Part model, mm, in its own coordinate system. Give positions to 0.01 mm unless a question says otherwise; leave off trailing zeros. Write each loop counter-clockwise with the first axis right and the second up, starting at its lowest first coordinate (ties: lowest second). Pieces come first, ordered by that corner, then holes. Notation, with made-up numbers: (11, 30) - (26, 30) arc R24 cw to (26, 66) - close; hole circle Ø11 at (22, 23.25). An arc over 180 degrees is marked (long way). Answer as a JSON object with one key per item and string values. Group by question number.
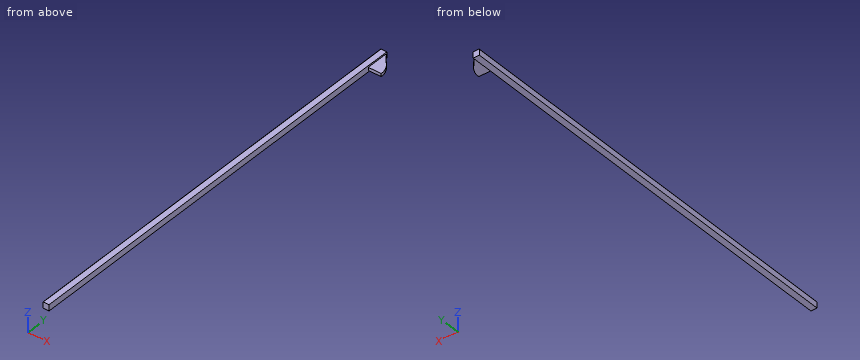
```python
from build123d import *

# Parameters (mm, degrees)
BOSS_EXTRUDE1_DEPTH = 0.220347005
SKETCH2_W           = 0.335173503
SKETCH2_H           = 31
BOSS_EXTRUDE2_DEPTH = 0.45
SKETCH3_W           = 0.45
SKETCH3_H           = 31
BOSS_EXTRUDE3_DEPTH = 0.114826497
FILLET1_R           = 0.025


with BuildPart() as part:
    # Sketch1 → Boss-Extrude1 (new body)
    with BuildSketch(Plane(origin=(0, 0, -0.110173503), x_dir=(-1, 0, 0), z_dir=(0, 0, -1))):
        with BuildLine():
            Line((-0.100899126, 1.3), (0.85, 1.3))
            Line((0.85, 1.3), (0.85, 2.9))
            Line((0.85, 2.9), (0.754271379, 2.9))
            add(Edge.make_bspline(
                [(0.754271379, 2.9), (0.756059912, 2.890829896), (0.757688053, 2.871605997), (0.754283259, 2.84011903), (0.73796652, 2.792795969), (0.697785469, 2.724539071), (0.638294458, 2.646987167), (0.561118331, 2.56007299), (0.469917194, 2.464054427), (0.370218593, 2.359510578), (0.26840655, 2.24717531), (0.17098544, 2.127849346), (0.083811745, 2.002312001), (0.011182268, 1.871255904), (-0.044647472, 1.735241835), (-0.08270041, 1.594693954), (-0.098810181, 1.47885747), (-0.102928932, 1.390139391), (-0.102161317, 1.330181827), (-0.100899126, 1.3)],
                knots=[0, 0, 0, 0, 0, 0, 0.066666667, 0.133333333, 0.2, 0.266666667, 0.333333333, 0.4, 0.466666667, 0.533333333, 0.6, 0.666666667, 0.733333333, 0.8, 0.866666667, 0.933333333, 1, 1, 1, 1, 1, 1], degree=5))
        make_face()
    extrude(amount=-BOSS_EXTRUDE1_DEPTH)

    # Sketch2 → Boss-Extrude2 (add)
    with BuildSketch(Plane(origin=(-0.85, 0, 0), x_dir=(0, 0, -1), z_dir=(1, 0, 0))):
        with Locations((-0.057413248, -12.5)):
            Rectangle(SKETCH2_W, SKETCH2_H)
    extrude(amount=-BOSS_EXTRUDE2_DEPTH)

    # Sketch3 → Boss-Extrude3 (add)
    with BuildSketch(Plane(origin=(0, 0, -0.110173503), x_dir=(-1, 0, 0), z_dir=(0, 0, -1))):
        with Locations((1.075, -12.5)):
            Rectangle(SKETCH3_W, SKETCH3_H)
    extrude(amount=BOSS_EXTRUDE3_DEPTH)

    # Fillet1
    fillet1_edges = [part.edges().sort_by_distance(p)[0] for p in [
        (-1.3, -12.5, 0.225),
    ]]
    fillet(fillet1_edges, radius=FILLET1_R)


solid = part.part
```
1) Drill centre lines: line 1 along X through (y, z) = (-24, -0.1); line 2 along X through (y, z) = (1.5, -0.05); line 3 along Y through (x, z) = (-0.7, 0). Where is each one in solid material? Low to high. Write a range as from..to.
2) Saw through at A-A (y = -1.5). List the corners of the cut face in (x, z) (3 decimals).
3) Drop a flat-ended pin along its axis: P1, Ø0.5, axis at x = -0.5, y = 2, coming from the +Z side. Give the stop position or say it passes through.
Checks:
{
 "1": {"line 1": "-1.3..-0.85", "line 2": "-1.3..0.09", "line 3": "1.3..2.73"},
 "2": {"outline": "(-1.3, -0.225) - (-0.85, -0.225) - (-0.85, 0.225) - (-1.275, 0.225) arc R0.025 ccw to (-1.3, 0.2) - close"},
 "3": {"P1": "z = 0.11"}
}
